Part model, mm, in its own coordinate system. A direction names the side the tool comes from. Coordinates: 2 decimals unless noted, no trailing zeros. Loops run counter-clockwise (first coordinate to the right, second up) from the corner with the lowest first, then second, coordinate; pieces in that order, holes last. Notation, with made-up numbers: M -37.75,-33 L -14.75,-33 A17 ccw -14.75,-22 Z; hole C 61.5,5.25 d1. An arc over 180 degrees is marked long. Answer as a JSON object with one key per item and string values. Group by question number.
1. Mould opens along Z. For faces 3 (the face through (37.43, -0.1, -39.35)), 4 (the face through (2.64, -1.34, -59.94)), 5 (the face through (1, 7.5, -1)) say: released by +Z, released by -Z, zero draft, split by the parting line, or undercut.
2. Saw through at A-A on x = 19.5. Write the cut outline in (y, z).
3. Drop flat-ended pins along their axis: pin 1 Ø8 at (x, z) = (35.36, 35.36) entering from -Y; pin 2 Ø8 at (y, z) = (5, 3.5) entering from +X; pin 3 Ø3 at (x, y) = (-3, 6) entering from -Z; pin 4 Ø2 at (x, y) = (27.5, -1.5) entering from -Z. Give the stop position or say it passes through.
4. Saw through at B-B on y = -3. Write the cut outline in (x, z).
5. Drill centre lines: L1, parallel to Z at x = 33, y = -0.5; L2, parallel to Z at x = 32, y = -5.5. Where is each one in solid material? Low to high.
6. Saw through at C-C on z = -52.5. Write the cut outline in (x, y), then the cut area to 3 significant figures.
7. 3-axis set-ups, long thin cutter, end or side, ignore diameter. For faces 1 (the face through (-55.645, 6.268, -12.356)), 2 (the face through (-37.43, -0.1, 39.35)): which of +Z, -Z, +X, -X, +Y, -Y reach the whole face in a straight line?
from build123d import *

# Parameters (mm, degrees)
SKETCH1_R            = 57
EXTRUDE4_DEPTH       = 7.5
EXTRUDE5_DEPTH       = 5
EXTRUDE5_DEPTH_BACK  = 7.5
SKETCH_R             = 60
SKETCH_R_2           = 57
M8_CLEARANCE_HOLE3_D = 9
CIRPATTERN1_COUNT    = 4


with BuildPart() as part:
    # Sketch1 → Extrude4 (new, symmetric)
    with BuildSketch(Plane(origin=(0, 0, 0), x_dir=(1, 0, 0), z_dir=(0, 1, 0))):
        with Locations(Location((0, 0, 0), (0, 0, 270))):
            Circle(SKETCH1_R)
    extrude(amount=EXTRUDE4_DEPTH, both=True)

    # Sketch → Extrude5 (add, two sides: drawn at the far end of the back side and taken through both)
    with BuildSketch(Plane(origin=(0, 0, 0), x_dir=(1, 0, 0), z_dir=(0, 1, 0)).offset(-EXTRUDE5_DEPTH_BACK)):
        with Locations(Location((0, 0, 0), (0, 0, 270))):
            Circle(SKETCH_R)
        with Locations(Location((0, 0, 0), (0, 0, 270))):
            Circle(SKETCH_R_2, mode=Mode.SUBTRACT)
    extrude(amount=EXTRUDE5_DEPTH + EXTRUDE5_DEPTH_BACK)

    # M8 Clearance Hole3 (through all)
    with Locations(Plane(origin=(0, 7.5, 0), x_dir=(1, 0, 0), z_dir=(0, 1, 0))):
        with Locations((-35.355339059, -35.355339059)):
            m8_clearance_hole3 = Hole(M8_CLEARANCE_HOLE3_D / 2)

    # CirPattern1: M8 Clearance Hole3 ×4 about axis
    cirpattern1_axis = Axis((0, 0, 0), (0, 1, 0))
    for i in range(1, CIRPATTERN1_COUNT):
        add(m8_clearance_hole3.rotate(cirpattern1_axis, i * 360 / CIRPATTERN1_COUNT), mode=Mode.SUBTRACT)


solid = part.part
Outcome:
{
 "1": {"face 3": "undercut", "face 4": "split by the parting line", "face 5": "zero draft"},
 "2": {"outline": "M -7.5,-56.74 L 5,-56.74 L 5,-53.56 L 7.5,-53.56 L 7.5,53.56 L 5,53.56 L 5,56.74 L -7.5,56.74 Z"},
 "3": {"pin 1": "passes through", "pin 2": "stops at x = 60", "pin 3": "stops at z = -59.97", "pin 4": "stops at z = -53.83"},
 "4": {"outline": "C 0,0 d120; hole C -35.36,-35.36 d9; hole C -35.36,35.36 d9; hole C 35.36,-35.36 d9; hole C 35.36,35.36 d9"},
 "5": {"L1": "z = -50.11 to -39.19, -31.52 to 31.52, 39.19 to 50.11", "L2": "z = -50.75 to -38.35, -32.36 to 32.36, 38.35 to 50.75"},
 "6": {"outline": "M -29.05,-7.5 L 29.05,-7.5 L 29.05,5 L 22.2,5 L 22.2,7.5 L -22.2,7.5 L -22.2,5 L -29.05,5 Z", "area": "837 mm²"},
 "7": {"face 1": "+Y", "face 2": "+Y, -Y"}
}
